```python
from build123d import *

# Parameters (mm, degrees)
SKETCH_4_R          = 8
CUT_EXTRUDE_1_DEPTH = 38.336309405
SKETCH_5_R          = 9
CUT_EXTRUDE_2_DEPTH = 0.8


with BuildPart() as part:
    # Эскиз1 → Повернуть1 (revolve)
    with BuildSketch(Plane.XY, mode=Mode.PRIVATE) as revolve_1_sk:
        with BuildLine():
            Line((-4, 25), (-2.94403514, 19.609934257))
            ThreePointArc((-2.94403514, 19.609934257), (-2.52454557, 18.565998224), (-1.75, 17.75))
            ThreePointArc((-1.75, 17.75), (0, 16), (1.75, 17.75))
            ThreePointArc((1.75, 17.75), (2.52454557, 18.565998224), (2.94403514, 19.609934257))
            Line((2.94403514, 19.609934257), (4, 25))
            Line((4, 25), (6, 25))
            Line((6, 25), (6, 0))
            Line((6, 0), (-6, 0))
            Line((-6, 0), (-6, 25))
            Line((-6, 25), (-4, 25))
        make_face()
    revolve(revolve_1_sk.sketch.rotate(Axis((-6, 0, 0), (1, 0, 0)), 90), axis=Axis((-6, 0, 0), (1, 0, 0)))

    # Эскиз4 → Вырез-Вытянуть1 (cut, through all)
    with BuildSketch(Plane.ZY.offset(6)):
        Circle(SKETCH_4_R)
    extrude(amount=-CUT_EXTRUDE_1_DEPTH, mode=Mode.SUBTRACT)

    # Эскиз5 → Вырез-Вытянуть2 (cut)
    with BuildSketch(Plane.ZY.offset(6)):
        Circle(SKETCH_5_R)
    cut_extrude_2 = extrude(amount=-CUT_EXTRUDE_2_DEPTH, mode=Mode.SUBTRACT)

    # Зеркальное отражение1: Вырез-Вытянуть2 across plane
    add(cut_extrude_2.mirror(Plane(origin=(0, 0, 0), x_dir=(0, 0, 1), z_dir=(1, 0, 0))), mode=Mode.SUBTRACT)


solid = part.part
```
Work out the finished part from the listing and answer in its coordinate system (mm). A direction names the side the tool comes from. Coordinates: 2 decimals unless noted, no trailing zeros. Loops run counter-clockwise (first coordinate to the right, second up) from the corner with the lowest first, then second, coordinate; pieces in that order, holes last. Notation, with made-up numbers: (73.25, 13.25) -> (109.25, 13.25) arc R27 cw to (109.25, 31.25) -> close; hole circle Ø6 at (36.25, 40). An arc over 180 degrees is marked (long way). Answer as CSV lines item,"result".
Q1. The part is cut by section C-C on x = 0. Write down the section's boundary in (y, z), and give its area (3 significant figures).
Findings:
outline,"circle Ø32 at (0, 0); hole circle Ø16 at (0, 0)"
area,"603 mm²"
Q2. For a pull along Y with two mould halves and no side action, classify faces 4 (the face through (-0.07, -7.81, -1.73)), 5 (the face through (-6, 11, 0)), 6 (the face through (-5.606, 8.923, -1.172)), 7 (the face through (-4.986, -7.509, 23.846)) as +Y half, -Y half, draft (parallel to the pull), parting line (faces both ways), or undercut.
Findings:
face 4,"undercut"
face 5,"draft"
face 6,"undercut"
face 7,"parting line"
Q3. The part is cut by section A-A on z = 0. Write down the section's boundary in (x, y), and give its area (3 significant figures).
Findings:
outline,"(-6, -25) -> (-4, -25) -> (-2.94, -19.61) arc R3 cw to (-1.75, -17.75) arc R1.75 cw to (1.75, -17.75) arc R3 cw to (2.94, -19.61) -> (4, -25) -> (6, -25) -> (6, -9) -> (5.2, -9) -> (5.2, -8) -> (-5.2, -8) -> (-5.2, -9) -> (-6, -9) -> close; (-6, 9) -> (-5.2, 9) -> (-5.2, 8) -> (5.2, 8) -> (5.2, 9) -> (6, 9) -> (6, 25) -> (4, 25) -> (2.94, 19.61) arc R3 cw to (1.75, 17.75) arc R1.75 cw to (-1.75, 17.75) arc R3 cw to (-2.94, 19.61) -> (-4, 25) -> (-6, 25) -> close"
area,"302 mm²"
Q4. Each of these flat-tipped pins is pushed along its axis until it touches: pin 1 (2 mm diameter, centred on y = -3.5, z = 7, fed in from +X); pin 2 (1 mm diameter, centred on x = -4, y = 19.5, fed in from +Z). Where does it stop, or does it pass through?
Findings:
pin 1,"stops at x = 5.2"
pin 2,"stops at z = 16.25"
Q5. Find the intervals of material crossed by probe 1 along X at (y, z) = (21, 13.5); probe 2 along Y at (x, z) = (5.85, 0); probe 3 along Z at (x, y) = (5, 15.5), in increasing order.
Findings:
probe 1,"x = -6 to -3.99, 3.99 to 6"
probe 2,"y = -25 to -9, 9 to 25"
probe 3,"z = -19.62 to 19.62"
Q6. A tool of negligible diameter and unlimited length cuts with its end or side. For faces 1 (the face through (5.014, -7.509, 23.846)), 2 (the face through (5.606, 8.923, -1.172)), 3 (the face through (-2.995, 19.399, -4.308)), from which of +Z, -Z, +X, -X, +Y, -Y can it reach the whole face along a straight path? Write none if from no direction.
Findings:
face 1,"+X, -X"
face 2,"+X"
face 3,"none"
